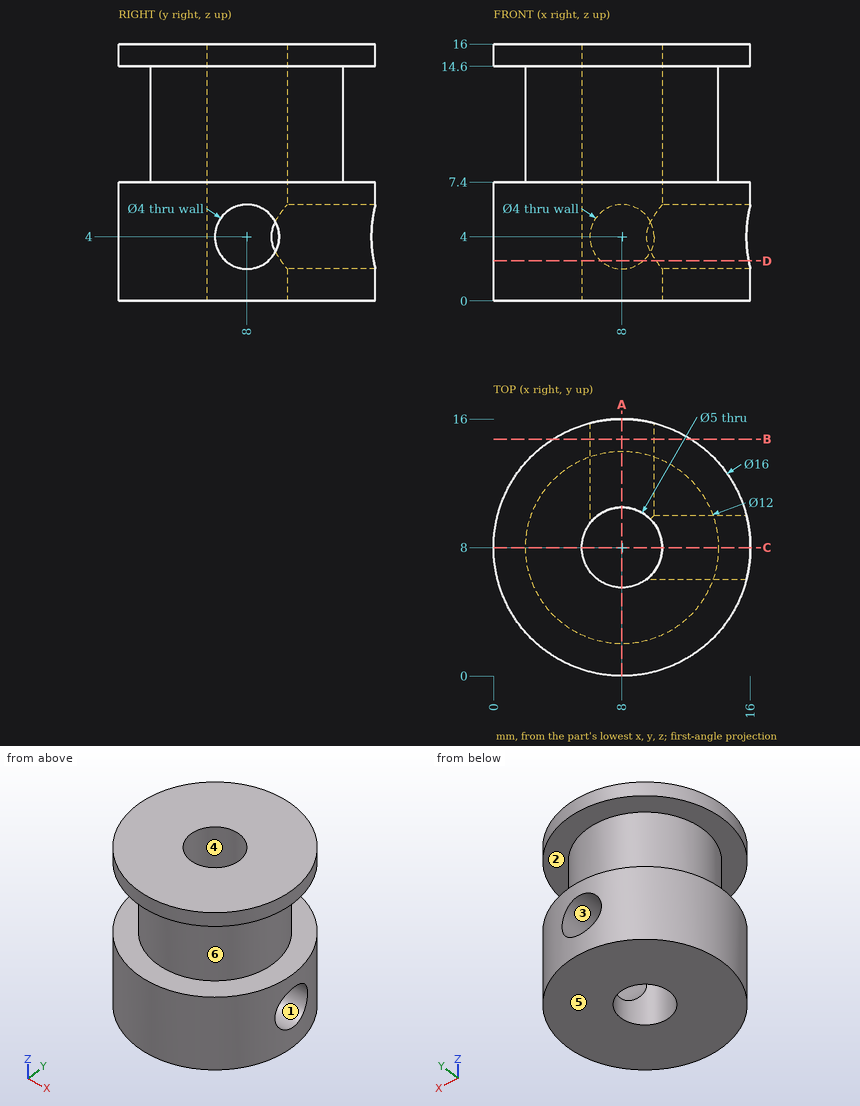
Geometry: see drawing. Coordinates: mm, zero at the bounding-box minimum. A direction names the side the tool comes from. Coordinates: 2 decimals unless noted, no trailing zeros. Loops run counter-clockwise (first coordinate to the right, second up) from the corner with the lowest first, then second, coordinate; pieces in that order, holes last.
Q1. Contact query for flat-ended pins moving along their axis: pin 1 (1 mm diameter, centred on y = 12.5, z = 9.5, fed in from -X); pin 2 (1.5 mm diameter, centred on x = 2, z = 9.5, fed in from -Y); pin 3 (1.5 mm diameter, centred on y = 11.5, z = 2.5, fed in from +X). Output: stop coordinate, or through.
Q2. Draft query along Y for the marked faces 4, 5 and 6. Return one class per face: +Y half, -Y half, draft (parallel to the pull), parting line (faces both ways), or undercut.
Q3. Material intervals for line 1 (Y direction, x = 8, z = 7.25); line 2 (Z direction, x = 2, y = 13); line 3 (Y direction, x = 7.75, z = 10.5), sorted ascending.
Q4. Set-up query: the marked faces 1, 2 and 3. Return all of +Z, -Z, +X, -X, +Y, -Y with unobstructed straight access to the full face (end or side cutting, diameter ignored); none if empty.
Q5. Cut plane D-D (z = 2.5). Output: boundary loops of the cut face in (x, y).
Q6. Cut plane A-A (x = 8). Output: boundary loops of the cut face in (y, z).
Q7. Cut plane B-B (y = 14.75). Output: boundary loops of the cut face in (x, z), then the cut area to 3 significant figures.
Working result:
1. pin 1: stops at x = 3.53
1. pin 2: stops at y = 5.1
1. pin 3: stops at x = 15.51
2. face 4: undercut
2. face 5: draft
2. face 6: parting line
3. line 1: y = 0 to 5.5, 10.5 to 16
3. line 2: z = 0 to 7.4, 14.6 to 16
3. line 3: y = 2.01 to 5.51, 10.49 to 13.99
4. face 1: +X
4. face 2: none
4. face 3: +Y
5. outline: (6.68, 10.12) - (6.68, 15.89) arc R8 ccw (long way) to (15.89, 6.68) - (10.12, 6.68) arc R2.5 cw (long way) to start; (9.32, 10.12) arc R2.5 cw to (10.12, 9.32) - (15.89, 9.32) arc R8 ccw to (9.32, 15.89) - close
6. outline: (0, 0) - (5.5, 0) - (5.5, 16) - (0, 16) - (0, 14.6) - (2, 14.6) - (2, 7.4) - (0, 7.4) - close; (10.5, 0) - (16, 0) - (16, 2) - (10.5, 2) - close; (10.5, 6) - (16, 6) - (16, 7.4) - (14, 7.4) - (14, 14.6) - (16, 14.6) - (16, 16) - (10.5, 16) - close
7. outline: (3.71, 0) - (12.29, 0) - (12.29, 7.4) - (3.71, 7.4) - close; (3.71, 14.6) - (12.29, 14.6) - (12.29, 16) - (3.71, 16) - close; hole circle Ø4 at (8, 4)
7. area: 63.0 mm2
